Design review of the part built by this model. Coordinates are the model's own, in mm. Face numbers are marked on the shaded views. A direction names the side the tool comes from. Round coordinates to 2 decimals unless told otherwise and drop trailing zeros. Write each loop counter-clockwise with the first axis right and the second up, starting at its lowest first coordinate (ties: lowest second). Pieces come first, ordered by that corner, then holes.
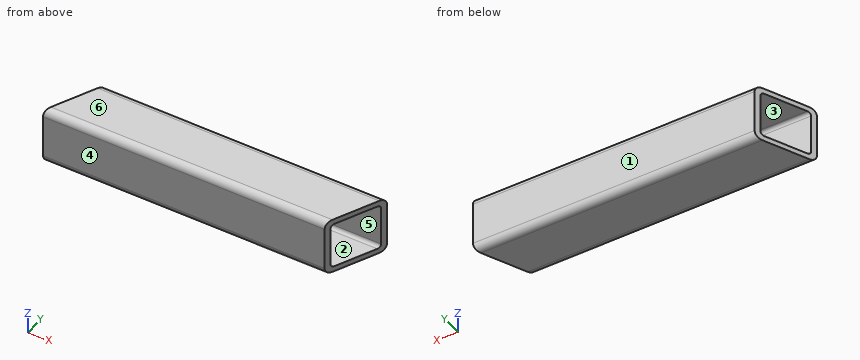
from build123d import *

# Parameters (mm, degrees)
F1_DEPTH = 1651
F3_DEPTH = 127


with BuildPart() as f1:
    # F0 (on Right) → F1 (new body)
    with BuildSketch(Plane.YZ):
        with BuildLine():
            Line((88.9, 0), (12.7, 0))
            ThreePointArc((12.7, 0), (3.719744, -3.719744), (0, -12.7))
            Line((0, -12.7), (0, -88.9))
            ThreePointArc((0, -88.9), (3.719744, -97.880256), (12.7, -101.6))
            Line((12.7, -101.6), (88.9, -101.6))
            ThreePointArc((88.9, -101.6), (97.880256, -97.880256), (101.6, -88.9))
            Line((101.6, -88.9), (101.6, -12.7))
            ThreePointArc((101.6, -12.7), (97.880256, -3.719744), (88.9, 0))
        make_face()
        with BuildLine():
            ThreePointArc((9.525, -15.875), (11.384872, -11.384872), (15.875, -9.525))
            Line((15.875, -9.525), (85.725, -9.525))
            ThreePointArc((85.725, -9.525), (90.215128, -11.384872), (92.075, -15.875))
            Line((92.075, -15.875), (92.075, -85.725))
            ThreePointArc((92.075, -85.725), (90.215128, -90.215128), (85.725, -92.075))
            Line((85.725, -92.075), (15.875, -92.075))
            ThreePointArc((15.875, -92.075), (11.384872, -90.215128), (9.525, -85.725))
            Line((9.525, -85.725), (9.525, -15.875))
        make_face(mode=Mode.SUBTRACT)
    extrude(amount=F1_DEPTH)

    # F2 (on Top) → F3 (cut)
    with BuildSketch(Plane.XY):
        Polygon((505.073142, 0), (1651, 0), (1651, 12.7), (1651, 88.9), (1651, 101.6), (552.45, 101.6), align=None)
        Polygon((0, 12.7), (0, 0), (47.376858, 101.6), (0, 101.6), (0, 88.9), align=None)
    extrude(amount=-F3_DEPTH, mode=Mode.SUBTRACT)


solid = f1.part
1) Add section A-A on z = -35. State the section outline as (x, y) points (3 decimals).
2) For line 1 along Y through (x, z) = (186, -53) (3 decimals); line 2 along Z through (x, y) = (232, 23) (3 decimals); line 3 along Y through (x, z) = (371, -12.5), list the stretches that pass through material, from the lowest coordinate up.
3) Add section C-C on x = 317.5. State the section outline as (y, z) points (3 decimals), and give its area (3 significant figures).
4) The part is to be moulded in two halves that separate along Z. For the marked faces 3, 4, 5 and 6, say which applies: pulls with the +Z half, pulls with the -Z half, needs draft (parallel to the pull), parting line crosses it, or undercut.
5) Add section B-B on y = 66.5. State the section outline as (x, z) points (3 decimals).
6) For the marked faces 1 and 2, list the 3-axis set-ups (+Z, -Z, +X, -X, +Y, -Y) from which the entire face can be reached by the end or side of a thin tool; tool diameter is ignored.
Computed:
1. outline: (0, 0) - (505.073, 0) - (509.515, 9.525) - (4.442, 9.525) - close; (42.935, 92.075) - (548.008, 92.075) - (552.45, 101.6) - (47.377, 101.6) - close
2. line 1: y = 0 to 9.525, 92.075 to 101.6
2. line 2: z = -101.6 to -92.075, -9.525 to 0
2. line 3: y = 0 to 10.5, 91.1 to 101.6
3. outline: (0, -88.9) arc R12.7 ccw to (12.7, -101.6) - (88.9, -101.6) arc R12.7 ccw to (101.6, -88.9) - (101.6, -12.7) arc R12.7 ccw to (88.9, 0) - (12.7, 0) arc R12.7 ccw to (0, -12.7) - close; hole (9.525, -85.725) arc R6.35 ccw to (15.875, -92.075) - (85.725, -92.075) arc R6.35 ccw to (92.075, -85.725) - (92.075, -15.875) arc R6.35 ccw to (85.725, -9.525) - (15.875, -9.525) arc R6.35 ccw to (9.525, -15.875) - close
3. area: 3,400 mm2
4. face 3: undercut
4. face 4: needs draft
4. face 5: undercut
4. face 6: pulls with the +Z half
5. outline: (31.009, -101.6) - (536.083, -101.6) - (536.083, -92.075) - (31.009, -92.075) - close; (31.009, -9.525) - (536.083, -9.525) - (536.083, 0) - (31.009, 0) - close
6. face 1: +Z, -Z, +X, -X, +Y
6. face 2: +X, -X
